Can you work these out from the drawing? Everything is in mm from the part's minimum corner. Round coordinates to 2 decimals unless told otherwise and drop trailing zeros. Loops run counter-clockwise (first coordinate to the right, second up) from the corner with the lowest first, then second, coordinate; pieces in that order, holes last. Notation, with made-up numbers: (-35, 41) - (-6, 41) arc R28 ccw to (-6, 71) - close; hole circle Ø6 at (-25.75, -30). An arc over 180 degrees is marked (long way). Answer as a JSON object with one key per item and string values. Group by question number.
1) I want a section at C-C, the plane x = 57. Please give me the cut outline in (y, z), then the cut area to 3 significant figures.
2) I want a section at B-B, the plane z = 41. Please give me the cut outline in (x, y), then the cut area to 3 significant figures.
3) Will these pins go through, and if not, where does the flat tip stop? P1, Ø5, axis at x = 3.048, z = 3.048, coming from the +Y side; P2, Ø0.8, axis at y = 0.5, z = 39, coming from the +X side; P3, Ø0.8, axis at x = 62.5, y = 1, coming from the +Z side.
4) If I drill on line 1 along X through (y, z) = (0.4, 3.5); line 2 along X through (y, z) = (0.9, 48); line 3 along Z through (x, y) = (70, 0.2), over which ranges is the centre line in solid material (lowest first)? Write a range as [from, to].
5) I want a section at A-A, the plane y = 0.4. Please give me the cut outline in (x, z).
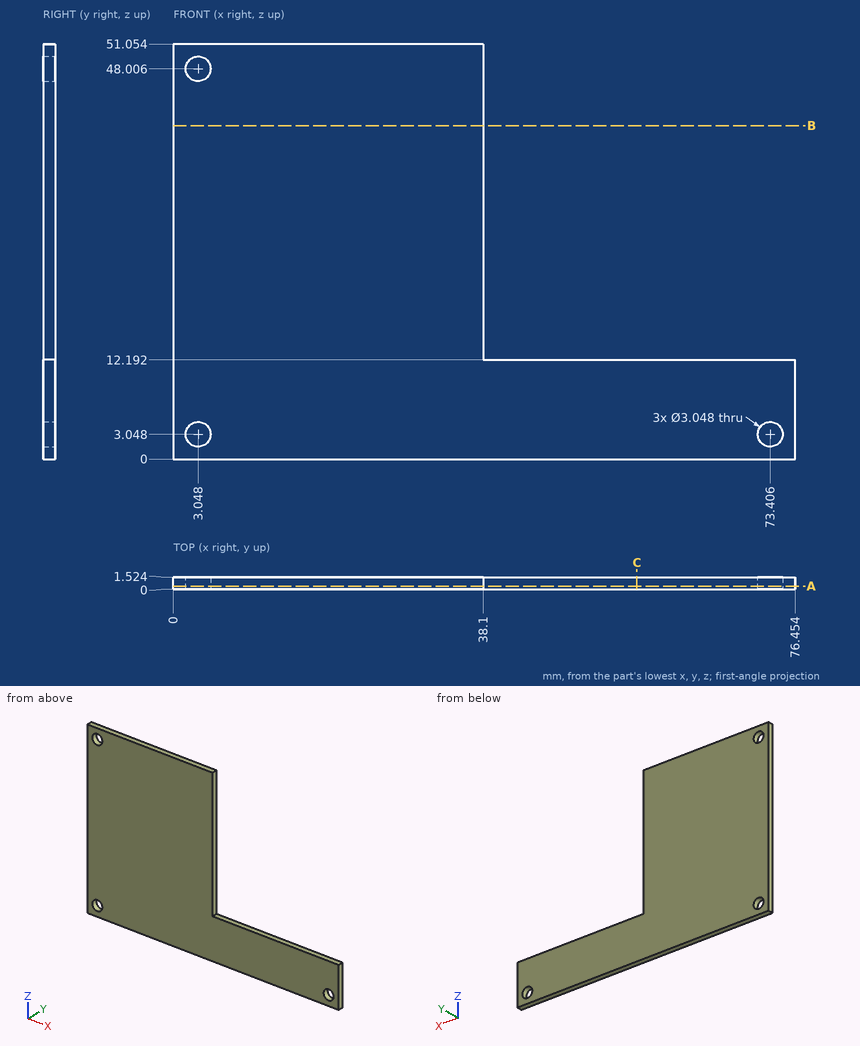
Outcome:
{
 "1": {"outline": "(0, 0) - (1.52, 0) - (1.52, 12.19) - (0, 12.19) - close", "area": "18.6 mm^2"},
 "2": {"outline": "(0, 0) - (38.1, 0) - (38.1, 1.52) - (0, 1.52) - close", "area": "58.1 mm^2"},
 "3": {"P1": "y = 1.52", "P2": "x = 38.1", "P3": "z = 12.19"},
 "4": {"line 1": "[0, 1.59], [4.5, 71.95], [74.86, 76.45]", "line 2": "[0, 1.52], [4.57, 38.1]", "line 3": "[0, 12.19]"},
 "5": {"outline": "(0, 0) - (76.45, 0) - (76.45, 12.19) - (38.1, 12.19) - (38.1, 51.05) - (0, 51.05) - close; hole circle Ø3.05 at (3.05, 3.05); hole circle Ø3.05 at (3.05, 48.01); hole circle Ø3.05 at (73.41, 3.05)"}
}
